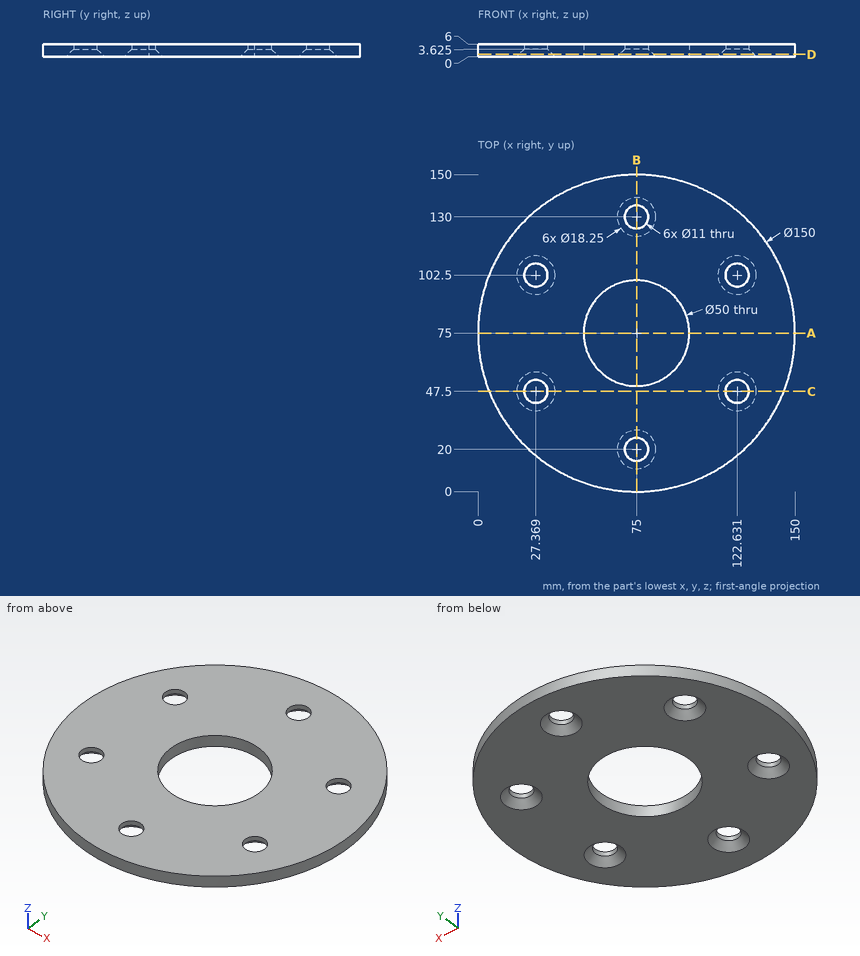
Geometry: see drawing. Coordinates: mm, zero at the bounding-box minimum. Round coordinates to 2 decimals unless told otherwise and drop trailing zeros. Write each loop counter-clockwise with the first axis right and the second up, starting at its lowest first coordinate (ties: lowest second). Pieces come first, ordered by that corner, then holes.
Item 1: Section query A-A (y = 75). Return loops of the section in (x, z).
Item 2: Section query B-B (x = 75). Return loops of the section in (y, z) (1 decimal).
Item 3: Pin query (flat end, axial travel): P1, Ø14.5, axis at x = 122.63, y = 47.5, coming from the -Z side (1 decimal); P2, Ø1.5, axis at x = 85.5, z = 2, coming from the +Y side; P3, Ø17.5, axis at x = 122.63, y = 102.5, coming from the -Z side (1 decimal); P4, Ø10, axis at x = 75, y = 130, coming from the +Z side. Return the tip coordinate at first contact, or that it passes through.
Item 4: Section query C-C (y = 47.5). Return loops of the section in (x, z) (1 decimal), plus the area to 3 significant figures.
Item 5: Section query D-D (z = 1.05). Give the number of separate pieces and of enclosed holes in the cut face, plus the area to 3 significant figures.
Item 6: Material intervals for L1, parallel to Y at x = 75, z = 5.55; L2, parallel to X at y = 47, z = 2.05 (1 decimal); L3, parallel to Y at x = 70, z = 4.3 (1 decimal), sorted ascending.
Completed:
1. outline: (0, 0) - (50, 0) - (50, 6) - (0, 6) - close; (100, 0) - (150, 0) - (150, 6) - (100, 6) - close
2. outline: (0, 0) - (10.9, 0) - (14.5, 3.6) - (14.5, 6) - (0, 6) - close; (25.5, 3.6) - (29.1, 0) - (50, 0) - (50, 6) - (25.5, 6) - close; (100, 0) - (120.9, 0) - (124.5, 3.6) - (124.5, 6) - (100, 6) - close; (135.5, 3.6) - (139.1, 0) - (150, 0) - (150, 6) - (135.5, 6) - close
3. P1: stops at z = 1.9
3. P2: stops at y = 149.36
3. P3: stops at z = 0.4
3. P4: passes through
4. outline: (5.2, 0) - (18.2, 0) - (21.9, 3.6) - (21.9, 6) - (5.2, 6) - close; (32.9, 3.6) - (36.5, 0) - (113.5, 0) - (117.1, 3.6) - (117.1, 6) - (32.9, 6) - close; (128.1, 3.6) - (131.8, 0) - (144.8, 0) - (144.8, 6) - (128.1, 6) - close
4. area: 679 mm2
5. separate pieces: 1
5. enclosed holes: 7
5. area: 14,500 mm2
6. L1: y = 0 to 14.5, 25.5 to 50, 100 to 124.5, 135.5 to 150
6. L2: x = 5.4 to 20.3, 34.4 to 115.6, 129.7 to 144.6
6. L3: y = 0.2 to 17.7, 22.3 to 50.5, 99.5 to 127.7, 132.3 to 149.8
